```python
from build123d import *

# Parameters (mm, degrees)
BOSS_EXTRUDE1_DEPTH = 180
SKETCH4_R           = 1.25
CUT_EXTRUDE1_DEPTH  = 5


with BuildPart() as part:
    # Sketch1 → Boss-Extrude1 (new body)
    with BuildSketch(Plane.XY):
        Polygon((3.770690633, -1.334875333), (3.041381265, 2.598076211), (-0.729309367, 3.932951544), (-3.770690633, 1.334875333), (-3.041381265, -2.598076211), (0.729309367, -3.932951544), align=None)
    extrude(amount=BOSS_EXTRUDE1_DEPTH)

    # Sketch4 → Cut-Extrude1 (cut)
    with BuildSketch(Plane(origin=(0, 0, 0), x_dir=(-1, 0, 0), z_dir=(0, 0, -1))):
        Circle(SKETCH4_R)
    cut_extrude1 = extrude(amount=-CUT_EXTRUDE1_DEPTH, mode=Mode.SUBTRACT)

    # Mirror1: Cut-Extrude1 across plane
    add(cut_extrude1.mirror(Plane.XY.offset(90)), mode=Mode.SUBTRACT)


solid = part.part
```
Could you check a few things on this model? Use its own coordinates, in mm. Give positions to 0.01 mm unless a question says otherwise; leave off trailing zeros. Loops run counter-clockwise (first coordinate to the right, second up) from the corner with the lowest first, then second, coordinate; pieces in that order, holes last. Notation, with made-up numbers: (58.25, 74) -> (98.25, 74) arc R24 ccw to (98.25, 93) -> close; hole circle Ø9 at (15, 31.5). An arc over 180 degrees is marked (long way). Put each result on its own line as item: value.
(1) Imagine slicing it at B-B on y = 0. Write out the boundary of the cut face in (x, z), plus the area to 3 significant figures.
Computed:
outline: (-3.52, 0) -> (-1.25, 0) -> (-1.25, 5) -> (1.25, 5) -> (1.25, 0) -> (3.52, 0) -> (3.52, 180) -> (1.25, 180) -> (1.25, 175) -> (-1.25, 175) -> (-1.25, 180) -> (-3.52, 180) -> close
area: 1,240 mm^2
(2) I'm going to push flat-ended pins straight in: pin 1 Ø4 at (y, z) = (-3, 29) entering from -X; pin 2 Ø2 at (y, z) = (-2.5, 112.5) entering from +X; pin 3 Ø1.5 at (x, z) = (-2, 87.5) entering from -Y. Where does each tip first touch, or does it pass through?
Computed:
pin 1: x = -3.34
pin 2: x = 3.58
pin 3: y = -3.23
(3) Please list where these lines run through material, in increasing order: probe 1 along Y at (x, z) = (0, 3.95); probe 2 along Z at (x, y) = (0.5, -0.75); probe 3 along X at (y, z) = (-0.75, 24). Write a range as [from, to].
Computed:
probe 1: [-3.67, -1.25], [1.25, 3.67]
probe 2: [5, 175]
probe 3: [-3.38, 3.66]
(4) Imagine slicing it at A-A on z = 132.5. Write out the boundary of the cut face in (x, y).
Computed:
outline: (-3.77, 1.33) -> (-3.04, -2.6) -> (0.73, -3.93) -> (3.77, -1.33) -> (3.04, 2.6) -> (-0.73, 3.93) -> close
(5) Thinking about a two-plate mould opening in Z: for faces 1 (the face through (-1, 1, 0)), 2 (the face through (-1, 1, 180)), 3 (the face through (-3.41, -0.6, 88.74)), which applies, pulls with the +Z half, pulls with the -Z half, needs draft (parallel to the pull), parting line crosses it, or undercut?
Computed:
face 1: pulls with the -Z half
face 2: pulls with the +Z half
face 3: needs draft
